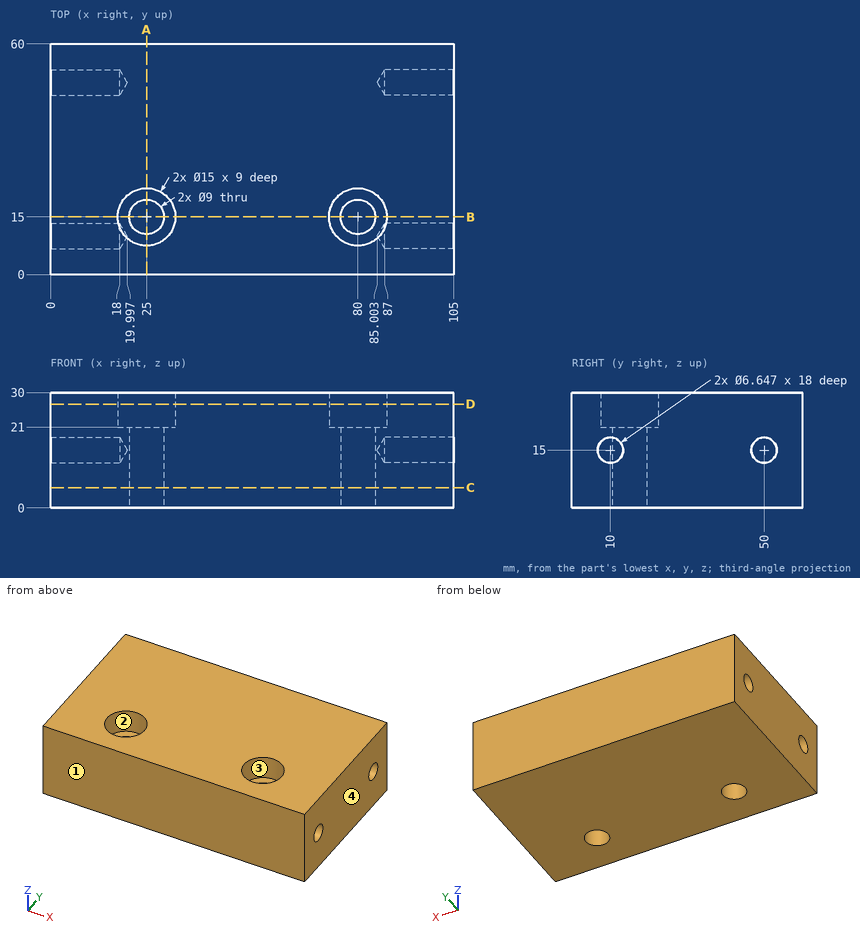
The figure shows three views and two pictorial views of one solid part (mm, origin at its lowest corner). Answer the questions. Give positions to 0.01 mm unless a question says otherwise; leave off trailing zeros. Write each loop counter-clockwise with the first axis right and the second up, starting at its lowest first coordinate (ties: lowest second). Pieces come first, ordered by that corner, then holes. Notation, with made-up numbers: M 67.25,16 L 82.25,16 A33 ccw 82.25,53 Z; hole C 8.5,-18.75 d11. An arc over 180 degrees is marked long. One line per item, written item: value. Start each with the question number.
(1) Flat-ended cylindrical pins translate along their axes: pin 1 Ø1.5 at (x, z) = (59, 13) entering from -Y; pin 2 Ø11.5 at (x, y) = (80, 15) entering from +Z; pin 3 Ø4 at (y, z) = (10, 15) entering from -X; pin 4 Ø8 at (x, y) = (25, 15) entering from -Z. Find the tip coordinate at first contact, or state that the pin passes through.
(2) Find section C-C (z = 5.25). Determine the outline of the cut face in (x, y).
(3) Determine the mould class of the marked faces 1, 2, 3 and 4 for opening direction X: pulls with the +X half, pulls with the -X half, needs draft (parallel to the pull), parting line crosses it, or undercut.
(4) Find section D-D (z = 27). Determine the outline of the cut face in (x, y).
(5) Find section B-B (y = 15). Determine the outline of the cut face in (x, z).
(6) Find section A-A (x = 25). Determine the outline of the cut face in (y, z), plus the area to 3 significant figures.
(7) Find the intervals of material crossed by line 1 (Y direction, x = 98.5, z = 15); line 2 (Z direction, x = 100.25, y = 50); line 3 (X direction, y = 15, z = 7), in increasing order.
Results below:
1. pin 1: stops at y = 0
1. pin 2: stops at z = 21
1. pin 3: stops at x = 18.8
1. pin 4: passes through
2. outline: M 0,0 L 105,0 L 105,60 L 0,60 Z; hole C 25,15 d9; hole C 80,15 d9
3. face 1: needs draft
3. face 2: undercut
3. face 3: undercut
3. face 4: pulls with the +X half
4. outline: M 0,0 L 105,0 L 105,60 L 0,60 Z; hole C 25,15 d15; hole C 80,15 d15
5. outline: M 0,0 L 20.5,0 L 20.5,21 L 17.5,21 L 17.5,30 L 0,30 Z; M 29.5,0 L 75.5,0 L 75.5,21 L 72.5,21 L 72.5,30 L 32.5,30 L 32.5,21 L 29.5,21 Z; M 84.5,0 L 105,0 L 105,30 L 87.5,30 L 87.5,21 L 84.5,21 Z
6. outline: M 0,0 L 10.5,0 L 10.5,21 L 7.5,21 L 7.5,30 L 0,30 Z; M 19.5,0 L 60,0 L 60,30 L 22.5,30 L 22.5,21 L 19.5,21 Z
6. area: 1,480 mm^2
7. line 1: y = 0 to 6.68, 13.32 to 46.68, 53.32 to 60
7. line 2: z = 0 to 11.68, 18.32 to 30
7. line 3: x = 0 to 20.5, 29.5 to 75.5, 84.5 to 105
